```python
from build123d import *

# Parameters (mm, degrees)
SKETCH_1_R      = 5
EXTRUDE_1_DEPTH = 60
SKETCH_2_R      = 4
EXTRUDE_2_DEPTH = 50


with BuildPart() as part:
    # 草图1 → 凸台-拉伸1 (new, symmetric)
    with BuildSketch(Plane(origin=(0, 0, 0), x_dir=(0, 0, -1), z_dir=(1, 0, 0))):
        Circle(SKETCH_1_R)
    extrude(amount=EXTRUDE_1_DEPTH, both=True)

    # 草图2 → 凸台-拉伸2 (add)
    with BuildSketch(Plane(origin=(0, 0, 0), x_dir=(1, 0, 0), z_dir=(0, 1, 0))):
        with Locations(Location((0, 0, 0), (0, 0, 90))):
            Circle(SKETCH_2_R)
    extrude(amount=EXTRUDE_2_DEPTH)


with BuildPart() as part_1:
    # Move Body 1: moved
    add(part.part.moved(Location((60, 0, 0))))


solid = part_1.part
```
Design review of the part built by this model. Coordinates are the model's own, in mm. A direction names the side the tool comes from. Give positions to 0.01 mm unless a question says otherwise; leave off trailing zeros. Order: outer loops, then holes, each group sorted by start corner. A loop starts at its lowest first (then second) coordinate and runs counter-clockwise, first axis right, second up. Notation, with made-up numbers: (17.5, 30) - (26.5, 30) arc R12 cw to (26.5, 39) - close; hole circle Ø6 at (48, -23). An arc over 180 degrees is marked (long way). Use a Markdown table: item, result. Add a question column.
(1) Add section C-C on y = 12. Give the boundary of the cut face in (x, z), then the cut area to 3 significant figures.
(2) Clearance check with flat-ended pins moving along their axes: P1, Ø1.5, axis at y = 17.5, z = 3, coming from the +X side; P2, Ø8, axis at x = 28, y = 1.5, coming from the -Z side; P3, Ø12, axis at x = 106, y = 12.5, coming from the -Z side; P4, Ø4, axis at y = 41, z = 3, coming from the -X side. State where each tip first meets the part, or that it passes through.
(3) Machinability: for faces 1 (the face through (120, 0, 0)), 2 (the face through (63.905, 26.171, 0.867)), 3 (the face through (60.84, -4.88, 1.08)), which of the approach directions +Z, -Z, +X, -X, +Y, -Y give a long, thin tool a straight path to every point of the face, cutting with its end or side? Answer none if there is none.
(4) Wall thickness on probe 1 along X at (y, z) = (41, -0.25); probe 2 along Z at (x, y) = (9, 0.5); probe 3 along X at (y, z) = (19, 2.75): over which ranges is each line inside the solid? List them lowest first. Write a range as [from, to].
(5) Add section D-D on x = 60. Give the boundary of the cut face in (y, z), then the cut area to 3 significant figures.
(6) Add section A-A on z = 0. Give the boundary of the cut face in (x, y), then the cut area to 3 significant figures.
(7) Add section B-B on x = 35. Give the boundary of the cut face in (y, z), then the cut area to 3 significant figures.
Report:
| question | item | result |
|---|---|---|
| 1 | outline | circle Ø8 at (60, 0) |
| 1 | area | 50.3 mm² |
| 2 | P1 | stops at x = 63.31 |
| 2 | P2 | stops at z = -5 |
| 2 | P3 | passes through |
| 2 | P4 | stops at x = 56.13 |
| 3 | face 1 | +Z, -Z, +X, +Y, -Y |
| 3 | face 2 | +Y |
| 3 | face 3 | none |
| 4 | probe 1 | x = [56.01, 63.99] |
| 4 | probe 2 | z = [-4.97, 4.97] |
| 4 | probe 3 | x = [57.1, 62.9] |
| 5 | outline | (3, -4) - (50, -4) - (50, 4) - (3, 4) arc R5 ccw (long way) to start |
| 5 | area | 443 mm² |
| 6 | outline | (0, -5) - (120, -5) - (120, 5) - (64, 5) - (64, 50) - (56, 50) - (56, 5) - (0, 5) - close |
| 6 | area | 1,560 mm² |
| 7 | outline | circle Ø10 at (0, 0) |
| 7 | area | 78.5 mm² |
